Part model, mm, in its own coordinate system. Face numbers are marked on the shaded views. A direction names the side the tool comes from. Coordinates: 2 decimals unless noted, no trailing zeros. Loops run counter-clockwise (first coordinate to the right, second up) from the corner with the lowest first, then second, coordinate; pieces in that order, holes last.
```python
from build123d import *

# Parameters (mm, degrees)
F1_DEPTH  = 25.4
F3_DEPTH  = 25.401
F5_DEPTH  = 9.780613
F6_R      = 6.35
F7_DEPTH  = 25.401
F8_R      = 6.35
F11_DEPTH = 9.780613


with BuildPart() as f1:
    # F0 (on Front) → F1 (new body)
    with BuildSketch(Plane.XZ):
        Polygon((0, 38.1), (0, 0), (71.12, 0), (71.12, 9.779613), (33.02, 9.779613), (33.02, 38.1), align=None)
    extrude(amount=F1_DEPTH)

    # F2 (on face) → F3 (cut, through all)
    with BuildSketch(Plane.XZ.offset(25.4)):
        with BuildLine():
            ThreePointArc((0, 23.861155), (16.80079, 38.095578), (33.02, 23.20187))
            Line((33.02, 23.20187), (33.02, 38.1))
            Line((33.02, 38.1), (0, 38.1))
            Line((0, 38.1), (0, 23.861155))
        make_face()
    extrude(amount=-F3_DEPTH, mode=Mode.SUBTRACT)

    # F4 (on face) → F5 (cut, through all)
    with BuildSketch(Plane.XY.offset(9.779613)):
        with BuildLine():
            ThreePointArc((61.019834, 0), (68.153419, -4.578181), (71.12, -12.518407))
            Line((71.12, -12.518407), (71.12, 0))
            Line((71.12, 0), (61.019834, 0))
        make_face()
        with BuildLine():
            ThreePointArc((71.12, -13.490307), (68.731865, -20.658356), (62.849611, -25.4))
            Line((62.849611, -25.4), (71.12, -25.4))
            Line((71.12, -25.4), (71.12, -13.490307))
        make_face()
    extrude(amount=-F5_DEPTH, mode=Mode.SUBTRACT)

    # F6 (on face) → F7 (cut, through all)
    with BuildSketch(Plane(origin=(0, 0, 0), x_dir=(-1, 0, 0), z_dir=(0, 1, 0))):
        with Locations((-16.468551, 21.455578)):
            Circle(F6_R)
    extrude(amount=-F7_DEPTH, mode=Mode.SUBTRACT)

    # F10 (on face) + F8 (on face) → F11 (cut, through all)
    with BuildSketch(Plane.XY.offset(9.779613)):
        with BuildLine():
            Line((58.540852, -6.708974), (57.118951, -6.681905))
            ThreePointArc((57.118951, -6.681905), (53.433667, -17.698736), (64.059799, -13.004357))
            ThreePointArc((64.059799, -13.004357), (62.484717, -8.81835), (58.540852, -6.708974))
        make_face()
    with BuildSketch(Plane.XY.offset(9.779613)):
        with Locations((44.713352, -12.77754)):
            Circle(F8_R)
    extrude(amount=-F11_DEPTH, mode=Mode.SUBTRACT)


solid = f1.part
```
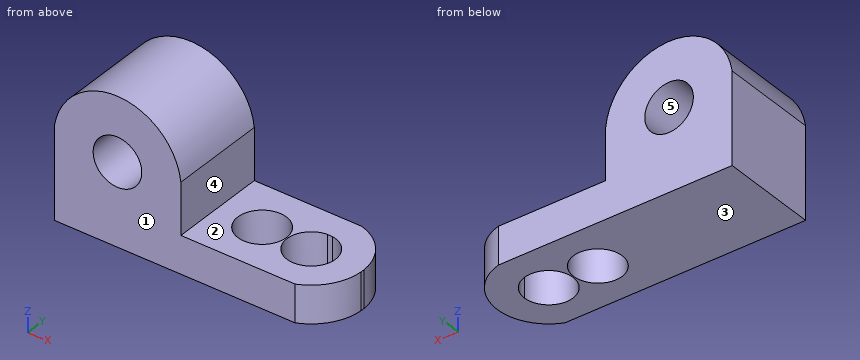
Q1. Mould opens along Z. For the marked faces 3, 4 and 5 say: released by +Z, released by -Z, zero draft, split by the parting line, or undercut.
Q2. Saw through at A-A (y = -10). List the corners of the cut face in (x, z), plus the area to 3 significant figures.
Q3. Saw through at B-B (x = 60). List the corners of the cut face in (y, z), plus the area to 3 significant figures.
Q4. Drop flat-ended pins along their axis: P1, Ø1, axis at y = -19, z = 34, coming from the +X side; P2, Ø10.5, axis at y = -14, z = 14, coming from the +X side; P3, Ø3, axis at y = -3, z = 12.5, coming from the +X side; P4, Ø8, axis at x = 62, y = -14.5, coming from the +Z side. Give the stop position or say it passes through.
Q5. Saw through at C-C (z = 25). List the corners of the cut face in (x, y), plus the area to 3 significant figures.
Q6. Tool access for the marked faces 1 and 2: list every direction of +Z, -Z, +X, -X, +Y, -Y with a clear straight run to the whole face (end or side of a thin tool).
Q7. Saw through at D-D (y = -23). List the corners of the cut face in (x, z).
Q8. Probe line 1 (X direction, y = -12.75, z = 4.5); line 2 (X direction, y = -13.5, z = 9.5); line 3 (Z direction, x = 17, y = -15.25). List the from-to ranges inside material, lowest first.
Checked values:
1. face 3: released by -Z
1. face 4: zero draft
1. face 5: undercut
2. outline: (0, 0) - (39, 0) - (39, 9.78) - (33.02, 9.78) - (33.02, 23.2) arc R16.64 ccw to (0, 23.86) - close; (50.42, 0) - (52.12, 0) - (52.12, 9.78) - (50.42, 9.78) - close; (63.3, 0) - (70.79, 0) - (70.79, 9.78) - (63.3, 9.78) - close; hole circle Ø12.7 at (16.47, 21.46)
2. area: 1,160 mm2
3. outline: (-25.4, 0) - (-18.93, 0) - (-18.93, 9.78) - (-25.4, 9.78) - close; (-7.08, 0) - (0, 0) - (0, 9.78) - (-7.08, 9.78) - close
3. area: 133 mm2
4. P1: stops at x = 27.95
4. P2: stops at x = 71.12
4. P3: stops at x = 33.02
4. P4: stops at z = 9.78
5. outline: (0.21, -25.4) - (11.2, -25.4) - (11.2, 0) - (0.21, 0) - close; (21.74, -25.4) - (32.73, -25.4) - (32.73, 0) - (21.74, 0) - close
5. area: 558 mm2
6. face 1: +Z, -Z, +X, -X, -Y
6. face 2: +Z, +X, +Y, -Y
7. outline: (0, 0) - (66.66, 0) - (66.66, 9.78) - (33.02, 9.78) - (33.02, 23.2) arc R16.64 ccw to (0, 23.86) - close; hole circle Ø12.7 at (16.47, 21.46)
8. line 1: x = 0 to 38.36, 51.06 to 51.36, 64.05 to 71.12
8. line 2: x = 0 to 38.4, 51.02 to 51.38, 64.04 to 71.12
8. line 3: z = 0 to 15.13, 27.78 to 38.09
